Work out the finished part from the listing and answer in its coordinate system (mm). A direction names the side the tool comes from. Coordinates: 2 decimals unless noted, no trailing zeros. Loops run counter-clockwise (first coordinate to the right, second up) from the corner with the lowest first, then second, coordinate; pieces in that order, holes last. Notation, with made-up numbers: (31, 87) -> (88, 87) arc R24 ccw to (88, 108) -> close; hole circle Ø3 at (13, -22). An arc over 180 degrees is marked (long way). Use a Markdown table: item, result. Add a question column.
```python
from build123d import *

# Parameters (mm, degrees)
SKETCH1_R                  = 15.875
EXTRUDE2_DEPTH             = 38.1
SKETCH2_R                  = 4.7625
CUT_EXTRUDE1_DEPTH         = 45.22263278
SKETCH8_R                  = 15.08125
CUT_EXTRUDE3_DEPTH         = 34.925
SKETCH9_R                  = 24.789766377
CUT_EXTRUDE4_DEPTH         = 2.54
SKETCH10_R                 = 26.9875
EXTRUDE3_DEPTH             = 20.32
SKETCH11_R                 = 25.4
CUT_EXTRUDE5_DEPTH         = 17.145
SKETCH12_R                 = 14.2875
CUT_EXTRUDE6_DEPTH         = 53.16477655
F_9_0_196_DIAMETER_HOLE1_D = 4.9784
CIRPATTERN1_COUNT          = 2
CIRPATTERN1_ANGLE          = 45
SKETCH17_R                 = 3.175
CUT_EXTRUDE7_DEPTH         = 86.064550432
CIRPATTERN2_COUNT          = 2


with BuildPart() as part:
    # Sketch1 → Extrude2 (new body)
    with BuildSketch(Plane(origin=(0, 0, 0), x_dir=(1, 0, 0), z_dir=(0, 1, 0))):
        with Locations(Location((0, 0, 0), (0, 0, 90))):
            Circle(SKETCH1_R)
    extrude(amount=EXTRUDE2_DEPTH)

    # Sketch2 → Cut-Extrude1 (cut, through all)
    with BuildSketch(Plane.XZ):
        with Locations(Location((0, 0, 0), (0, 0, 270))):
            Circle(SKETCH2_R)
    extrude(amount=-CUT_EXTRUDE1_DEPTH, mode=Mode.SUBTRACT)

    # Sketch8 → Cut-Extrude3 (cut)
    with BuildSketch(Plane(origin=(0, 38.1, 0), x_dir=(-1, 0, 0), z_dir=(0, 1, 0))):
        with Locations(Location((0, 0, 0), (0, 0, 90))):
            Circle(SKETCH8_R)
    extrude(amount=-CUT_EXTRUDE3_DEPTH, mode=Mode.SUBTRACT)

    # Sketch9 → Cut-Extrude4 (cut)
    with BuildSketch(Plane(origin=(0, 38.1, 0), x_dir=(-1, 0, 0), z_dir=(0, 1, 0))):
        Circle(SKETCH9_R)
    extrude(amount=-CUT_EXTRUDE4_DEPTH, mode=Mode.SUBTRACT)

    # Sketch10 → Extrude3 (add)
    with BuildSketch(Plane(origin=(0, 35.56, 0), x_dir=(-1, 0, 0), z_dir=(0, 1, 0))):
        with Locations(Location((0, 0, 0), (0, 0, 90))):
            Circle(SKETCH10_R)
    extrude(amount=EXTRUDE3_DEPTH)

    # Sketch11 → Cut-Extrude5 (cut)
    with BuildSketch(Plane(origin=(0, 55.88, 0), x_dir=(-1, 0, 0), z_dir=(0, 1, 0))):
        with Locations(Location((0, 0, 0), (0, 0, 90))):
            Circle(SKETCH11_R)
    extrude(amount=-CUT_EXTRUDE5_DEPTH, mode=Mode.SUBTRACT)

    # Sketch12 → Cut-Extrude6 (cut, through all)
    with BuildSketch(Plane(origin=(0, 35.56, 0), x_dir=(-1, 0, 0), z_dir=(0, 1, 0))):
        with Locations(Location((0, 0, 0), (0, 0, 90))):
            Circle(SKETCH12_R)
    extrude(amount=CUT_EXTRUDE6_DEPTH, mode=Mode.SUBTRACT)

    # #9 (0.196) Diameter Hole1 (through all)
    with Locations(Plane(origin=(-7.776127346, 55.88, -18.773232101), x_dir=(0, 0, 1), z_dir=(0, 1, 0))):
        with Locations((0, 0)):
            f_9_0_196_diameter_hole1 = Hole(F_9_0_196_DIAMETER_HOLE1_D / 2)

    # CirPattern1: #9 (0.196) Diameter Hole1 ×2 about axis
    cirpattern1_axis = Axis((0, 83.588580262, 0), (0, -1, 0))
    for i in range(1, CIRPATTERN1_COUNT):
        add(f_9_0_196_diameter_hole1.rotate(cirpattern1_axis, i * CIRPATTERN1_ANGLE / (CIRPATTERN1_COUNT - 1)), mode=Mode.SUBTRACT)

    # Sketch17 → Cut-Extrude7 (cut, through all)
    with BuildSketch(Plane(origin=(41.153091309, 43.18, 0), x_dir=(0, 0, -1), z_dir=(1, 0, 0))):
        Circle(SKETCH17_R)
    extrude(amount=-CUT_EXTRUDE7_DEPTH, mode=Mode.SUBTRACT)

    # Sketch20 → #10-32 Tapped Hole1 (revolve, cut)
    with BuildSketch(Plane(origin=(11.175940885, 0, 0.036350046), x_dir=(0, 0, -1), z_dir=(1, 0, 0))):
        Polygon((0, 0), (0, 13.252917848), (2.0193, 12.0396), (2.0193, 0), align=None)
    f_10_32_tapped_hole1 = revolve(axis=Axis((11.175940885, -6.35, 0.036350046), (0, 1, 0)), mode=Mode.SUBTRACT)

    # CirPattern2: #10-32 Tapped Hole1 ×2 about axis
    cirpattern2_axis = Axis((0, 0, 0), (0, 1, 0))
    for i in range(1, CIRPATTERN2_COUNT):
        add(f_10_32_tapped_hole1.rotate(cirpattern2_axis, i * 360 / CIRPATTERN2_COUNT), mode=Mode.SUBTRACT)


solid = part.part
```
Item 1: Find the intervals of material crossed by probe 1 along Y at (x, z) = (-26.2, 0) (3 decimals); probe 2 along Y at (x, z) = (0.5, 14.5) (3 decimals); probe 3 along X at (y, z) = (49, 0), in increasing order.
Item 2: Given pin 1 (4 mm diameter, centred on x = 7.78, z = -18.77, fed in from -Y); pin 2 (6 mm diameter, centred on y = 23, z = 1.5, fed in from +X) (3 decimals); pin 3 (10 mm diameter, centred on x = -15, y = 31, fed in from -Z); pin 4 (6 mm diameter, centred on x = 8.5, y = 9, fed in from -Z), each flat-ended and moving along its own axis, determine where each tip first touches the part or whether it passes through.
Item 3: Section D-D (z = 0) is taken. Count the separate pieces of the cut face and the enclosed holes in it, then the cut area to 3 significant figures.
Item 4: For a pull along X with two mould halves and no side action, classify faces 1 (the face through (-11, 38.735, 11)), 2 (the face through (26.11, 40.08, 0.69)), 3 (the face through (0.663, 19.594, -15.067)), 4 (the face through (18.24, 45.58, -19.89)) as +X half, -X half, draft (parallel to the pull), parting line (faces both ways), or undercut.
Item 5: Section B-B (y = 45.5) is taken. Determine the outline of the cut face in (x, z) (1 decimal), then the cut area to 3 significant figures.
Item 6: Section A-A (x = 0) is taken. Determine the outline of the cut face in (y, z) (1 decimal), then the cut area to 3 significant figures.
Item 7: For faces 5 (the face through (-12.22, 35.56, 7.75)), 6 (the face through (15.497, 17.531, 3.441)), 7 (the face through (-15.456, 47.428, -20.157)), 8 (the face through (-26.08, 40.08, 0.69)), determine the directions among +Z, -Z, +X, -X, +Y, -Y from which every point of the face is accessible in a straight line to the end or side of a thin tool.
Output:
| question | item | result |
|---|---|---|
| 1 | probe 1 | y = 35.56 to 40.005, 46.355 to 55.88 |
| 1 | probe 2 | y = 0 to 3.175, 35.56 to 38.735 |
| 1 | probe 3 | x = -26.99 to -25.4, 25.4 to 26.99 |
| 2 | pin 1 | passes through |
| 2 | pin 2 | stops at x = 15.875 |
| 2 | pin 3 | stops at z = -23.68 |
| 2 | pin 4 | stops at z = -14.89 |
| 3 | separate pieces | 6 |
| 3 | enclosed holes | 0 |
| 3 | area | 211 mm2 |
| 4 | face 1 | undercut |
| 4 | face 2 | draft |
| 4 | face 3 | undercut |
| 4 | face 4 | parting line |
| 5 | outline | (-26.9, -2.2) arc R27 ccw to (26.9, -2.2) -> (25.3, -2.2) arc R25.4 cw to (-25.3, -2.2) -> close; (-26.9, 2.2) -> (-25.3, 2.2) arc R25.4 cw to (25.3, 2.2) -> (26.9, 2.2) arc R27 ccw to start |
| 5 | area | 247 mm2 |
| 6 | outline | (0, -15.9) -> (35.6, -15.9) -> (35.6, -27) -> (55.9, -27) -> (55.9, -25.4) -> (38.7, -25.4) -> (38.7, -14.3) -> (35.6, -14.3) -> (35.6, -15.1) -> (3.2, -15.1) -> (3.2, -4.8) -> (0, -4.8) -> close; (0, 4.8) -> (3.2, 4.8) -> (3.2, 15.1) -> (35.6, 15.1) -> (35.6, 14.3) -> (38.7, 14.3) -> (38.7, 25.4) -> (55.9, 25.4) -> (55.9, 27) -> (35.6, 27) -> (35.6, 15.9) -> (0, 15.9) -> close |
| 6 | area | 257 mm2 |
| 7 | face 5 | none |
| 7 | face 6 | -Y |
| 7 | face 7 | +Y |
| 7 | face 8 | +X, -X |
